The listing builds one solid part. Answer for the finished solid, in the listing's coordinates (mm). A direction names the side the tool comes from. Coordinates: 2 decimals unless noted, no trailing zeros. Loops run counter-clockwise (first coordinate to the right, second up) from the corner with the lowest first, then second, coordinate; pieces in that order, holes last. Notation, with made-up numbers: (60, 35) - (110, 35) arc R10 cw to (110, 43) - close; hole circle Ø1 at (-15.75, 59). An arc over 180 degrees is marked (long way). Put each result on its own line as item: value.
```python
from build123d import *

# Parameters (mm, degrees)
F0_R     = 1.375
F0_R_2   = 1.75
F0_W     = 7
F0_H     = 5
F0_W_2   = 21.2
F0_H_2   = 43.2
F0_W_3   = 9.2
F0_H_3   = 33.2
F2_DEPTH = 1
F1_R     = 3
F1_R_2   = 1.5
F1_R_3   = 2.5
F1_R_4   = 1.75
F3_DEPTH = 2
F4_R     = 4


with BuildPart() as f2:
    # F0 (on Top) → F2 (new body)
    with BuildSketch(Plane.XY):
        with BuildLine():
            Line((-104.7829951048, -4.2856363673), (-119.2829951048, -4.2856363673))
            Line((-119.2829951048, -4.2856363673), (-119.2829951048, -34.2856363673))
            Line((-119.2829951048, -34.2856363673), (-104.7829951048, -34.2856363673))
            Line((-104.7829951048, -34.2856363673), (-104.7829951048, -29.2856363673))
            Line((-104.7829951048, -29.2856363673), (-109.2829951048, -29.2856363673))
            ThreePointArc((-109.2829951048, -29.2856363673), (-112.8185290107, -27.8211702732), (-114.2829951048, -24.2856363673))
            Line((-114.2829951048, -24.2856363673), (-114.2829951048, -14.2856363673))
            ThreePointArc((-114.2829951048, -14.2856363673), (-112.8185290107, -10.7501024614), (-109.2829951048, -9.2856363673))
            Line((-109.2829951048, -9.2856363673), (-104.7829951048, -9.2856363673))
            Line((-104.7829951048, -9.2856363673), (-104.7829951048, -4.2856363673))
        make_face()
        with Locations((-115.7829951048, -30.7856363673)):
            Circle(F0_R, mode=Mode.SUBTRACT)
        with Locations((-115.7829951048, -7.7856363673)):
            Circle(F0_R, mode=Mode.SUBTRACT)
        Polygon((-119.2829951048, -34.2856363673), (-119.2829951048, -4.2856363673), (-123.2829951048, 8.9143636327), (-123.2829951048, -34.2856363673), align=None)
        with BuildLine():
            Line((-104.7829951048, 23.2143636327), (-104.7829951048, -4.2856363673))
            Line((-104.7829951048, -4.2856363673), (-97.7829951048, -4.2856363673))
            Line((-97.7829951048, -4.2856363673), (-97.7829951048, 23.2143636327))
            ThreePointArc((-97.7829951048, 23.2143636327), (-101.2829951048, 26.7143636327), (-104.7829951048, 23.2143636327))
        make_face()
        with Locations((-101.2829951048, 23.2143636327)):
            Circle(F0_R_2, mode=Mode.SUBTRACT)
        with Locations((-101.2829951048, -6.7856363673)):
            Rectangle(F0_W, F0_H)
        with Locations((-133.8829951048, -12.6856363673)):
            Rectangle(F0_W_2, F0_H_2)
        with Locations((-141.9829951048, -27.7856363673)):
            Circle(F0_R_2, mode=Mode.SUBTRACT)
        with Locations((-125.7829951048, -27.7856363673)):
            Circle(F0_R_2, mode=Mode.SUBTRACT)
        with Locations((-133.8829951048, -12.6856363673)):
            Rectangle(F0_W_3, F0_H_3, mode=Mode.SUBTRACT)
        with Locations((-141.9829951048, 2.4143636327)):
            Circle(F0_R_2, mode=Mode.SUBTRACT)
        with Locations((-125.7829951048, 2.4143636327)):
            Circle(F0_R_2, mode=Mode.SUBTRACT)
        Polygon((-54.2829951048, -4.2856363673), (-97.7829951048, -4.2856363673), (-97.7829951048, -9.2856363673), (-88.7829951048, -9.2856363673), (-88.7829951048, -29.2856363673), (-97.7829951048, -29.2856363673), (-97.7829951048, -34.2856363673), (-54.2829951048, -34.2856363673), align=None)
        with Locations((-57.7829951048, -30.7856363673)):
            Circle(F0_R, mode=Mode.SUBTRACT)
        with BuildLine():
            ThreePointArc((-64.2829951048, -9.2856363673), (-60.7474611989, -10.7501024614), (-59.2829951048, -14.2856363673))
            Line((-59.2829951048, -14.2856363673), (-59.2829951048, -24.2856363673))
            ThreePointArc((-59.2829951048, -24.2856363673), (-60.7474611989, -27.8211702732), (-64.2829951048, -29.2856363673))
            Line((-64.2829951048, -29.2856363673), (-84.7829951048, -29.2856363673))
            Line((-84.7829951048, -29.2856363673), (-84.7829951048, -9.2856363673))
            Line((-84.7829951048, -9.2856363673), (-64.2829951048, -9.2856363673))
        make_face(mode=Mode.SUBTRACT)
        with Locations((-57.7829951048, -7.7856363673)):
            Circle(F0_R, mode=Mode.SUBTRACT)
        with Locations((-101.2829951048, -31.7856363673)):
            Rectangle(F0_W, F0_H)
        with BuildLine():
            Line((-97.7829951048, -34.2856363673), (-104.7829951048, -34.2856363673))
            Line((-104.7829951048, -34.2856363673), (-104.7829951048, -37.7856363673))
            ThreePointArc((-104.7829951048, -37.7856363673), (-101.2829951048, -41.2856363673), (-97.7829951048, -37.7856363673))
            Line((-97.7829951048, -37.7856363673), (-97.7829951048, -34.2856363673))
        make_face()
        with Locations((-101.2829951048, -37.7856363673)):
            Circle(F0_R_2, mode=Mode.SUBTRACT)
    extrude(amount=-F2_DEPTH)

    # F1 (on Top) → F3 (join)
    with BuildSketch(Plane.XY):
        with Locations((-115.7829951048, -7.7856363673)):
            Circle(F1_R)
        with Locations((-115.7829951048, -7.7856363673)):
            Circle(F1_R_2, mode=Mode.SUBTRACT)
        with Locations((-115.7829951048, -30.7856363673)):
            Circle(F1_R)
        with Locations((-115.7829951048, -30.7856363673)):
            Circle(F1_R_2, mode=Mode.SUBTRACT)
        with Locations((-57.7829951048, -7.7856363673)):
            Circle(F1_R)
        with Locations((-57.7829951048, -7.7856363673)):
            Circle(F1_R_2, mode=Mode.SUBTRACT)
        with Locations((-57.7829951048, -30.7856363673)):
            Circle(F1_R)
        with Locations((-57.7829951048, -30.7856363673)):
            Circle(F1_R_2, mode=Mode.SUBTRACT)
        with Locations((-141.9829951048, 2.4143636327)):
            Circle(F1_R_3)
        with Locations((-141.9829951048, 2.4143636327)):
            Circle(F1_R_4, mode=Mode.SUBTRACT)
        with Locations((-141.9829951048, -27.7856363673)):
            Circle(F1_R_3)
        with Locations((-141.9829951048, -27.7856363673)):
            Circle(F1_R_4, mode=Mode.SUBTRACT)
        with Locations((-125.7829951048, 2.4143636327)):
            Circle(F1_R_3)
        with Locations((-125.7829951048, 2.4143636327)):
            Circle(F1_R_4, mode=Mode.SUBTRACT)
        with Locations((-125.7829951048, -27.7856363673)):
            Circle(F1_R_3)
        with Locations((-125.7829951048, -27.7856363673)):
            Circle(F1_R_4, mode=Mode.SUBTRACT)
    extrude(amount=F3_DEPTH)

    # F4
    f4_edges = [f2.edges().sort_by_distance(p)[0] for p in [
        (-144.482995, 8.914364, -0.5),
        (-123.282995, 8.914364, -0.5),
        (-119.282995, -4.285636, -0.5),
        (-54.282995, -4.285636, -0.5),
        (-97.782995, -4.285636, -0.5),
        (-104.782995, -4.285636, -0.5),
        (-144.482995, -34.285636, -0.5),
        (-54.282995, -34.285636, -0.5),
        (-97.782995, -34.285636, -0.5),
        (-104.782995, -34.285636, -0.5),
    ]]
    fillet(f4_edges, radius=F4_R)


solid = f2.part
```
1) The part is cut by section D-D (x = -101). Give the vertices of the cut face in (y, z), and give its area (3 significant figures).
Found:
outline: (-41.27, -1) - (-39.51, -1) - (-39.51, 0) - (-41.27, 0) - close; (-36.06, -1) - (-29.29, -1) - (-29.29, 0) - (-36.06, 0) - close; (-9.29, -1) - (21.49, -1) - (21.49, 0) - (-9.29, 0) - close; (24.94, -1) - (26.7, -1) - (26.7, 0) - (24.94, 0) - close
area: 41.1 mm^2
2) Straight lines are drawn through the part: L1, parallel to X at y = 2.5, z = 0.05; L2, parallel to X at y = -23, z = -0.35; L3, parallel to Y at x = -93.5, z = -0.05. For each, find the intervals that lie inside material, in ascending order. Write a range as [from, to].
Found:
L1: x = [-144.48, -143.73], [-140.24, -139.48], [-128.28, -127.53], [-124.04, -123.28]
L2: x = [-144.48, -138.48], [-129.28, -114.28], [-88.78, -84.78], [-59.28, -54.28]
L3: y = [-34.29, -29.29], [-9.29, -4.29]
3) The part is cut by section A-A (y = -22.5). Give the vertices of the cut face in (x, z).
Found:
outline: (-144.48, -1) - (-138.48, -1) - (-138.48, 0) - (-144.48, 0) - close; (-129.28, -1) - (-114.28, -1) - (-114.28, 0) - (-129.28, 0) - close; (-88.78, -1) - (-84.78, -1) - (-84.78, 0) - (-88.78, 0) - close; (-59.28, -1) - (-54.28, -1) - (-54.28, 0) - (-59.28, 0) - close
4) For faces 4 (the face through (-54.922, -29.885, 0.986)), 5 (the face through (-112.86, -10.79, -0.49)), 6 (the face through (-143.28, -33.145, -0.507)), determine the directions among +Z, -Z, +X, -X, +Y, -Y from which every point of the face is accessible in a straight line to the end or side of a thin tool.
Found:
face 4: +Z
face 5: +Z, -Z
face 6: +Z, -Z, -X, -Y
5) The part is cut by section B-B (x = -71). Give the vertices of the cut face in (y, z), and give its area (3 significant figures).
Found:
outline: (-34.29, -1) - (-29.29, -1) - (-29.29, 0) - (-34.29, 0) - close; (-9.29, -1) - (-4.29, -1) - (-4.29, 0) - (-9.29, 0) - close
area: 10.0 mm^2
6) The part is cut by section C-C (z = 0.7). State how many separate pieces and enclosed holes the cut face has, and give its area (3 significant figures).
Found:
separate pieces: 8
enclosed holes: 8
area: 125 mm^2
7) For a pull along X with two mould halves and no side action, classify faces 1 (the face through (-121.267, 2.262, -0.493)), 2 (the face through (-144, 2, 2)), 3 (the face through (-55.42, -5.49, -0.51)) as pulls with the +X half, pulls with the -X half, needs draft (parallel to the pull), parting line crosses it, or undercut.
Found:
face 1: undercut
face 2: needs draft
face 3: pulls with the +X half
8) Each of these flat-tipped pins is pushed along its axis until it touches: pin 1 (0.8 mm diameter, centred on x = -133, z = -0.5, fed in from +Y); pin 2 (0.8 mm diameter, centred on x = -78.5, z = -0.5, fed in from -Y); pin 3 (0.8 mm diameter, centred on x = -70, z = -0.5, fed in from +Y). Where does it stop, or does it pass through?
Found:
pin 1: stops at y = 8.91
pin 2: stops at y = -34.29
pin 3: stops at y = -4.29
